The listing builds one solid part. Answer for the finished solid, in the listing's coordinates (mm). A direction names the side the tool comes from. Coordinates: 2 decimals unless noted, no trailing zeros. Order: outer loops, then holes, each group sorted by start corner. A loop starts at its lowest first (then second) coordinate and runs counter-clockwise, first axis right, second up. Notation, with made-up numbers: (-36.5, 81) -> (-7.5, 81) arc R7 ccw to (-7.5, 91) -> close; hole circle Ø10 at (-14.75, 30.5). An arc over 180 degrees is marked (long way). One line per question, with ' | ' between items.
from build123d import *

# Parameters (mm, degrees)
CYLINDER005_R          = 2.5
CYLINDER005_DEPTH      = 27
CYLINDER004_R          = 10
CYLINDER004_DEPTH      = 10
LINEAREXTRUDE003_DEPTH = 15


with BuildPart() as cylinder005:
    # cylinder005 → cylinder005 (new body)
    with BuildSketch(Plane.XY.offset(-1)):
        Circle(CYLINDER005_R)
    extrude(amount=CYLINDER005_DEPTH)


with BuildPart() as cylinder004:
    # cylinder004 → cylinder004 (new body)
    with BuildSketch(Plane.XY.offset(15)):
        Circle(CYLINDER004_R)
    extrude(amount=CYLINDER004_DEPTH)


with BuildPart() as pinion:
    # union004 → LinearExtrude003 (new body)
    with BuildSketch(Plane(origin=(0, 0, 0), x_dir=(0, 1, 0), z_dir=(0, 0, 1))):
        Polygon((0.711931, -4.306123), (1.370771, -4.143733), (1.502069, -4.540636), (1.530367, -4.602072), (1.641751, -4.771632), (1.871155, -5.020002), (2.245545, -5.309618), (2.782207, -5.596589), (3.025427, -5.468937), (3.094113, -4.864255), (3.068442, -4.391617), (2.994354, -4.061731), (2.918082, -3.873743), (2.883597, -3.815555), (2.631538, -3.482032), (3.139447, -3.032064), (3.440155, -3.322487), (3.493763, -3.363735), (3.671187, -3.46211), (3.989737, -3.575421), (4.455834, -3.657875), (5.064387, -3.662577), (5.220426, -3.436516), (5.000234, -2.869177), (4.757857, -2.462607), (4.53895, -2.204938), (4.384052, -2.073928), (4.326475, -2.038431), (3.948292, -1.860249), (4.188912, -1.225786), (4.590143, -1.343197), (4.656779, -1.354807), (4.859597, -1.359461), (5.194318, -1.311756), (5.645345, -1.168159), (6.186377, -0.889514), (6.219486, -0.616832), (5.76086, -0.216806), (5.357304, 0.030555), (5.043726, 0.156979), (4.845688, 0.200998), (4.77821, 0.205671), (4.36054, 0.187693), (4.278749, 0.861305), (4.688584, 0.943805), (4.752983, 0.964491), (4.934732, 1.054624), (5.208943, 1.252418), (5.541575, 1.58917), (5.891142, 2.087328), (5.793738, 2.344162), (5.201743, 2.485233), (4.729457, 2.516719), (4.393046, 2.482935), (4.197235, 2.429879), (4.135314, 2.402658), (3.773841, 2.192639), (3.388376, 2.751081), (3.712928, 3.01459), (3.760337, 3.062835), (3.879381, 3.227107), (4.030263, 3.529677), (4.168298, 3.982437), (4.246318, 4.585986), (4.040715, 4.768136), (3.45097, 4.617935), (3.018149, 4.426332), (2.735972, 4.240079), (2.587247, 4.102103), (2.545069, 4.049224), (2.322601, 3.695276), (1.721767, 4.010618), (1.886685, 4.394771), (1.906243, 4.459522), (1.93531, 4.6603), (1.928298, 4.99833), (1.840114, 5.463378), (1.628715, 6.034052), (1.362012, 6.099788), (0.909622, 5.692724), (0.61542, 5.321926), (0.452121, 5.025874), (0.384552, 4.834585), (0.371779, 4.768162), (0.339281, 4.351371), (-0.339281, 4.351371), (-0.371779, 4.768162), (-0.384552, 4.834585), (-0.452121, 5.025874), (-0.61542, 5.321926), (-0.909622, 5.692724), (-1.362012, 6.099788), (-1.628715, 6.034052), (-1.840114, 5.463378), (-1.928298, 4.99833), (-1.93531, 4.6603), (-1.906243, 4.459522), (-1.886685, 4.394771), (-1.721767, 4.010618), (-2.322601, 3.695276), (-2.545069, 4.049224), (-2.587247, 4.102103), (-2.735972, 4.240079), (-3.018149, 4.426332), (-3.45097, 4.617935), (-4.040715, 4.768136), (-4.246318, 4.585986), (-4.168298, 3.982437), (-4.030263, 3.529677), (-3.879381, 3.227107), (-3.760337, 3.062835), (-3.712928, 3.01459), (-3.388376, 2.751081), (-3.773841, 2.192638), (-4.135314, 2.402658), (-4.197235, 2.429879), (-4.393046, 2.482935), (-4.729457, 2.516719), (-5.201743, 2.485233), (-5.793738, 2.344162), (-5.891142, 2.087328), (-5.541575, 1.58917), (-5.208943, 1.252418), (-4.934732, 1.054624), (-4.752983, 0.964491), (-4.688584, 0.943805), (-4.278749, 0.861305), (-4.36054, 0.187693), (-4.77821, 0.205671), (-4.845688, 0.200998), (-5.043726, 0.156979), (-5.357304, 0.030555), (-5.76086, -0.216806), (-6.219486, -0.616832), (-6.186377, -0.889514), (-5.645345, -1.168159), (-5.194318, -1.311756), (-4.859597, -1.359461), (-4.656779, -1.354807), (-4.590143, -1.343197), (-4.188912, -1.225786), (-3.948292, -1.860249), (-4.326475, -2.038431), (-4.384052, -2.073928), (-4.53895, -2.204938), (-4.757857, -2.462607), (-5.000234, -2.869177), (-5.220426, -3.436516), (-5.064387, -3.662577), (-4.455834, -3.657875), (-3.989737, -3.575421), (-3.671187, -3.46211), (-3.493763, -3.363735), (-3.440155, -3.322487), (-3.139447, -3.032064), (-2.631537, -3.482032), (-2.883597, -3.815555), (-2.918082, -3.873743), (-2.994354, -4.061731), (-3.068442, -4.391617), (-3.094113, -4.864255), (-3.025427, -5.468937), (-2.782207, -5.596589), (-2.245545, -5.309618), (-1.871155, -5.020002), (-1.641751, -4.771632), (-1.530367, -4.602072), (-1.502069, -4.540636), (-1.370771, -4.143733), (-0.71193, -4.306122), (-0.780122, -4.71858), (-0.783616, -4.78613), (-0.763789, -4.98803), (-0.676085, -5.31456), (-0.47917, -5.74499), (-0.137342, -6.24849), (0.137342, -6.24849), (0.47917, -5.74499), (0.676085, -5.31456), (0.763789, -4.98803), (0.783616, -4.78613), (0.780122, -4.71858), align=None)
    extrude(amount=LINEAREXTRUDE003_DEPTH)

    # union005: union cylinder004
    add(cylinder004.part)

    # difference004: cut cylinder005
    add(cylinder005.part, mode=Mode.SUBTRACT)


solid = pinion.part
Item 1: Find the intervals of material crossed by L1, parallel to X at y = 0, z = 9.25; L2, parallel to Y at x = -4.5, z = 13.5; L3, parallel to Z at x = 4.25, y = -7.5, in increasing order.
Computed values:
L1: x = -4.35 to -2.5, 2.5 to 6.25 | L2: y = -4.24 to -3.18, -1.91 to -0.35, 0.35 to 1.91, 3.18 to 4.24 | L3: z = 15 to 25
Item 2: For faces 4 (the face through (-5, 0, 15)), 5 (the face through (0, 3, 0)), determine the directions among +Z, -Z, +X, -X, +Y, -Y from which every point of the face is accessible in a straight line to the end or side of a thin tool.
Computed values:
face 4: -Z | face 5: -Z, +X, -X, +Y, -Y
Item 3: Determine the mould class of faces 1 (the face through (-0.54, -2.44, 12.32)), 2 (the face through (2, -2, 25)), 3 (the face through (-2.17, -9.76, 19.93)) for opening direction X: pulls with the +X half, pulls with the -X half, needs draft (parallel to the pull), parting line crosses it, or undercut.
Computed values:
face 1: undercut | face 2: needs draft | face 3: parting line crosses it
Item 4: Section A-A, the plane y = -7.5 is taken. Give the vertices of the cut face in (x, z).
Computed values:
outline: (-6.61, 15) -> (6.61, 15) -> (6.61, 25) -> (-6.61, 25) -> close
Item 5: Section B-B, the plane x = 6.75 is taken. Give the vertices of the cut face in (y, z).
Computed values:
outline: (-7.38, 15) -> (7.38, 15) -> (7.38, 25) -> (-7.38, 25) -> close
Item 6: Each of these flat-tipped pins is pushed along its axis until it touches: pin 1 Ø6 at (x, z) = (2.5, 8.5) entering from +Y; pin 2 Ø4 at (x, y) = (6.5, 5.5) entering from -Z; pin 3 Ø5 at (y, z) = (7.5, 7.5) entering from -X. Where does it stop, or does it pass through?
Computed values:
pin 1: stops at y = 6.22 | pin 2: stops at z = 15 | pin 3: stops at x = -2.5
